Verification items for the finished model (mm, model axes). Coordinates: 2 decimals unless noted, no trailing zeros. Loops run counter-clockwise (first coordinate to the right, second up) from the corner with the lowest first, then second, coordinate; pieces in that order, holes last. Notation, with made-up numbers: (-3, 73.25) - (38, 73.25) arc R19 cw to (38, 85.25) - close; hole circle Ø8 at (13.5, 21.5). An arc over 180 degrees is marked (long way). Answer as CSV lines item,"result". Start each with the question number.
1. Material ranges on line 1 (Z direction, x = 19, y = 14.5); line 2 (Z direction, x = 51, y = 16); line 3 (Z direction, x = 50.5, y = 26), recorded low to high. Write a range as [from, to].
2. Cross-section at B-B (x = 11.5). Enter the section's corners in (y, z), plus the area to 3 significant figures.
3. Gauge pin test, flat ends, axial feed: P1, Ø6, axis at x = 23.5, z = 8.5, coming from the +Y side; P2, Ø4, axis at x = 2, z = 3.5, coming from the -Y side; P3, Ø3.5, axis at x = 2.5, y = 62.5, coming from the +Z side; P4, Ø1.5, axis at y = 9.5, z = 11.5, coming from the -X side. Record the tip position at first contact, or that the pin passes through.
4. Cross-section at C-C (z = 15). Enter the section's corners in (x, y).
5. Cross-section at A-A (y = 42.5). Enter the section's corners in (x, z).
Autodesk Inventor part; units mm, degrees
ref_plane "Płaszczyzna konstrukcyjna1" through (51.3468, 0, 6.6391) normal (-0.7236, 0, 0.6902) x (0.6902, 0, 0.7236)
ref_plane "YZ Plane" through (0, 0, 0) normal (1, 0, 0) x (0, 1, 0)
ref_plane "XZ Plane" through (0, 0, 0) normal (0, 1, 0) x (-1, 0, 0)
sketch "Szkic1" plane through (0, 0, 0) normal (0, 1, 0) x (-1, 0, 0)
  arc A0 (-57.7209, 16.9104) -> (-41.8849, 0) centre (-30, 27) ccw
  line L0 (-41.8849, 0) -> (-4, 0)
  line L1 (-4, 0) -> (-4, 3)
  line L2 (-57.7209, 16.9104) -> (-54.5041, 16.9104)
  line L3 (-54.5041, 16.9104) -> (-41.2361, 3)
  line L4 (-41.2361, 3) -> (-4, 3)
  line L5 (-4, 1.5) -> (-4, 3)
  dimension "d3" = 27
  dimension "d4" = 29.5
  dimension "d8" = 37.8849
  dimension "d9" = 37.2361
  dimension "d10" = 19.2234
extrude "Wyciągnięcie proste1" add sketch "Szkic1" along normal blind 72
sketch "Szkic3" plane through (4, 0, 0) normal (-1, 0, 0) x (0, 0, 1)
  line L0 (0, 0) -> (3, 0)
  line L1 (3, 0) -> (3, 72)
  line L2 (0, 72) -> (3, 72)
  line L3 (0, 0) -> (0, 72)
  line L4 (1.5, 5) -> (4.5, 5)
  line L5 (4.5, 5) -> (4.5, 11)
  line L6 (4.5, 11) -> (1.5, 11)
  line L7 (1.5, 11) -> (1.5, 5)
  line L8 (0, 0) -> (0, 72)
  line L9 (0, 36) -> (-11, 36)
  line L10 (1.5, 31) -> (4.5, 31)
  line L11 (4.5, 31) -> (4.5, 41)
  line L12 (4.5, 41) -> (1.5, 41)
  line L13 (1.5, 41) -> (1.5, 31)
  line L14 (1.5, 67) -> (4.5, 67)
  line L15 (4.5, 67) -> (4.5, 61)
  line L16 (4.5, 61) -> (1.5, 61)
  line L17 (1.5, 61) -> (1.5, 67)
  point P0 (1.5, 36)
  point P1 (0, 36)
  dimension "d15" = 3
  dimension "d16" = 6
  dimension "d17" = 4.5
  dimension "d18" = 5
  dimension "d19" = 3
  dimension "d20" = 10
  dimension "d21" = 4.5
extrude "Wyciągnięcie proste2" add sketch "Szkic3" along normal blind 4 contours L4 L7 L6 L1 | L1 L6 L5 L4 | L10 L13 L12 L1 | L1 L12 L11 L10 | L14 L15 L16 L1 | L1 L16 L17 L14
sketch "Szkic4" plane through (54.5041, 0, 16.9104) normal (-0.7236, 0, 0.6902) x (0.6902, 0, 0.7236)
  line L0 (-19.2234, 0) -> (0, 0)
  line L1 (0, 0) -> (0, 72)
  line L2 (-19.2234, 72) -> (0, 72)
  line L3 (-19.2234, 0) -> (-19.2234, 72)
  line L4 (-19.2234, 36) -> (0, 36)
  circle A0 centre (-7, 18) radius 1.6
  circle A1 centre (-7, 54) radius 1.6
  point P0 (-49.8554, 0)
  point P1 (-9.6117, 36)
  dimension "d26" = 3.2
  dimension "d27" = 36
  dimension "d34" = 7
extrude "Wyciągnięcie proste3" cut sketch "Szkic4" against normal through all contours A0 | A1
ref_plane "Płaszczyzna konstrukcyjna1" through (51.3468, 0, 6.6391) normal (-0.7236, 0, 0.6902) x (0.6902, 0, 0.7236)
sketch "Szkic5" plane through (51.3468, 0, 6.6391) normal (-0.7236, 0, 0.6902) x (0.6902, 0, 0.7236)
  circle A0 centre (2.6117, 54) radius 1.6
  circle A1 centre (2.6117, 18) radius 1.6
  line L0 (-9.6117, 0) -> (9.6117, 0)
  line L1 (9.6117, 0) -> (9.6117, 72)
  line L2 (-9.6117, 72) -> (9.6117, 72)
  line L3 (-9.6117, 0) -> (-9.6117, 72)
  circle A2 centre (2.6117, 54) radius 1.6
  circle A3 centre (2.6117, 54) radius 3
  circle A4 centre (2.6117, 18) radius 1.6
  circle A5 centre (2.6117, 18) radius 3
  point P0 (-40.2437, 0)
  dimension "d30" = 6
  dimension "d31" = 6
extrude "Wyciągnięcie proste4" cut sketch "Szkic5" along normal blind 3.3 contours A0 | A1 | A3 | A5
fillet "Zaokrąglenie3" radius 4 1 edges at (41.2361, 36, 3)
sketch "Szkic6" plane through (0, 0, 0) normal (-1, 0, 0) x (0, 0, 1)
  line L0 (4.5, 11) -> (1.5, 11)
  line L1 (1.5, 11) -> (1.5, 5)
  line L2 (1.5, 5) -> (4.5, 5)
  line L3 (4.5, 5) -> (4.5, 11)
  line L4 (4.5, 41) -> (1.5, 41)
  line L5 (1.5, 41) -> (1.5, 31)
  line L6 (1.5, 31) -> (4.5, 31)
  line L7 (4.5, 31) -> (4.5, 41)
  line L8 (4.5, 67) -> (1.5, 67)
  line L9 (1.5, 67) -> (1.5, 61)
  line L10 (1.5, 61) -> (4.5, 61)
  line L11 (4.5, 61) -> (4.5, 67)
  line L12 (1.7, 61.2) -> (1.7, 66.8)
  line L13 (1.7, 66.8) -> (4.3, 66.8)
  line L14 (4.3, 66.8) -> (4.3, 61.2)
  line L15 (4.3, 61.2) -> (1.7, 61.2)
  line L16 (4.3, 40.8) -> (1.7, 40.8)
  line L17 (1.7, 40.8) -> (1.7, 31.2)
  line L18 (1.7, 31.2) -> (4.3, 31.2)
  line L19 (4.3, 31.2) -> (4.3, 40.8)
  line L20 (4.3, 10.8) -> (1.7, 10.8)
  line L21 (1.7, 10.8) -> (1.7, 5.2)
  line L22 (1.7, 5.2) -> (4.3, 5.2)
  line L23 (4.3, 5.2) -> (4.3, 10.8)
  point P0 (0, 0)
  dimension "d36" = 0.2
  dimension "d37" = 0.2
  dimension "d38" = 0.2
extrude "Wyciągnięcie proste5" cut sketch "Szkic6" against normal up to surface (4 mm away)
fillet "Zaokrąglenie4" radius 1 9 edges at (4, 8, 1.7) (4, 36, 1.7) (4, 64, 1.7) (4, 36, 3) (4, 8, 3) (4, 64, 3) (4, 64, 4.3) (4, 36, 4.3) (4, 8, 4.3)
properties part number "pokrywka_baterii"
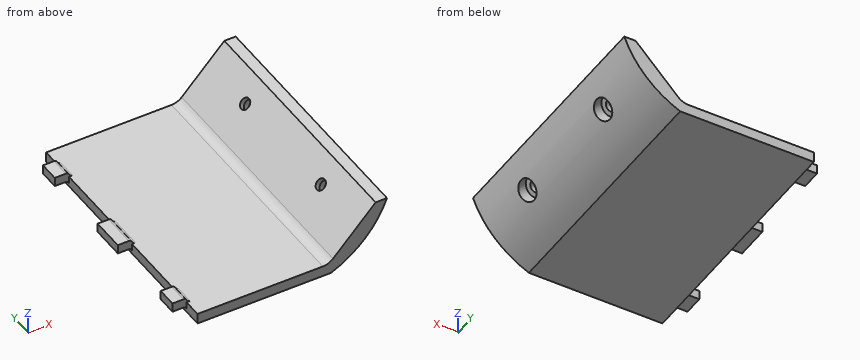
Values follow:
1,line 1,"z = [0, 3]"
1,line 2,"z = [6.28, 7.49], [11.06, 13.24]"
1,line 3,"z = [5.79, 12.71]"
2,outline,"(0, 0) - (72, 0) - (72, 3) - (0, 3) - close"
2,area,"216 mm²"
3,P1,"passes through"
3,P2,"stops at y = 5.2"
3,P3,"stops at z = 4.3"
3,P4,"stops at x = 48.63"
4,outline,"(52.68, 0) - (56.95, 0) - (56.95, 72) - (52.68, 72) - close"
5,outline,"(4, 0) - (41.88, 0) arc R29.5 ccw to (57.72, 16.91) - (54.5, 16.91) - (42.42, 4.24) arc R4 cw to (39.52, 3) - (4, 3) - close"
